```python
from build123d import *

# Parameters (mm, degrees)
SKETCH1_R               = 60
SKETCH1_R_2             = 2.5
SKETCH1_R_3             = 3
BOSS_EXTRUDE1_DEPTH     = 3
CUT_EXTRUDE1_DEPTH      = 85.905830189
CUT_EXTRUDE1_DEPTH_BACK = 85.905830189
SKETCH2_R               = 3


with BuildPart() as part:
    # Sketch1 → Boss-Extrude1 (new body)
    with BuildSketch(Plane(origin=(0, 0, 0), x_dir=(1, 0, 0), z_dir=(0, 1, 0))):
        with Locations(Location((0, 0, 0), (0, 0, 270))):
            Circle(SKETCH1_R)
        with Locations(Location((-24.748737342, -24.748737342, 0), (0, 0, 270))):
            Circle(SKETCH1_R_2, mode=Mode.SUBTRACT)
        with Locations(Location((24.748737342, -24.748737342, 0), (0, 0, 270))):
            Circle(SKETCH1_R_2, mode=Mode.SUBTRACT)
        with Locations(Location((24.748737342, 24.748737342, 0), (0, 0, 270))):
            Circle(SKETCH1_R_2, mode=Mode.SUBTRACT)
        with Locations(Location((-24.748737342, 24.748737342, 0), (0, 0, 270))):
            Circle(SKETCH1_R_2, mode=Mode.SUBTRACT)
        with Locations(Location((-25, -43.301270189, 0), (0, 0, 270))):
            Circle(SKETCH1_R_3, mode=Mode.SUBTRACT)
        with Locations(Location((25, -43.301270189, 0), (0, 0, 270))):
            Circle(SKETCH1_R_3, mode=Mode.SUBTRACT)
        with Locations(Location((50, 0, 0), (0, 0, 270))):
            Circle(SKETCH1_R_3, mode=Mode.SUBTRACT)
        with Locations(Location((25, 43.301270189, 0), (0, 0, 270))):
            Circle(SKETCH1_R_3, mode=Mode.SUBTRACT)
        with Locations(Location((-25, 43.301270189, 0), (0, 0, 270))):
            Circle(SKETCH1_R_3, mode=Mode.SUBTRACT)
        with Locations(Location((-50, 0, 0), (0, 0, 270))):
            Circle(SKETCH1_R_3, mode=Mode.SUBTRACT)
    extrude(amount=BOSS_EXTRUDE1_DEPTH)

    # Sketch2 → Cut-Extrude1 (cut, two sides: drawn at the far end of the back side and taken through both)
    with BuildSketch(Plane(origin=(0, 3, 0), x_dir=(1, 0, 0), z_dir=(0, 1, 0)).offset(-CUT_EXTRUDE1_DEPTH_BACK)):
        with Locations(Location((0, 0, 0), (0, 0, 270))):
            Circle(SKETCH2_R)
    extrude(amount=CUT_EXTRUDE1_DEPTH + CUT_EXTRUDE1_DEPTH_BACK, mode=Mode.SUBTRACT)


solid = part.part
```
The model under review builds one solid part; all positions refer to its coordinate system, in mm. Round coordinates to 2 decimals unless told otherwise and drop trailing zeros. Order: outer loops, then holes, each group sorted by start corner. A loop starts at its lowest first (then second) coordinate and runs counter-clockwise, first axis right, second up.
(1) Take a section at B-B, the plane y = 0.55. Count the separate pieces of the cut face and the enclosed holes in it, plus the area to 3 significant figures.
Working result:
separate pieces: 1
enclosed holes: 11
area: 11,000 mm2
(2) Take a section at A-A, the plane z = 0. State the section outline as (x, y) points, plus the area to 3 significant figures.
Working result:
outline: (-60, 0) - (-53, 0) - (-53, 3) - (-60, 3) - close; (-47, 0) - (-3, 0) - (-3, 3) - (-47, 3) - close; (3, 0) - (47, 0) - (47, 3) - (3, 3) - close; (53, 0) - (60, 0) - (60, 3) - (53, 3) - close
area: 306 mm2
(3) Take a section at C-C, the plane x = -50. State the section outline as (y, z) points.
Working result:
outline: (0, -33.17) - (3, -33.17) - (3, -3) - (0, -3) - close; (0, 3) - (3, 3) - (3, 33.17) - (0, 33.17) - close
(4) Mouldability with a two-part tool opening along Z and no side actions: class faces 1 (the face through (2.64, 1.48, -59.94)), 2 (the face through (-24.1, 1.48, -40.44)), 3 (the face through (1, 0, 12)) as released by +Z, released by -Z, zero draft, split by the parting line, or undercut.
Working result:
face 1: split by the parting line
face 2: undercut
face 3: zero draft
(5) Take a section at D-D, the plane x = 12. State the section outline as (y, z) points.
Working result:
outline: (0, -58.79) - (3, -58.79) - (3, 58.79) - (0, 58.79) - close
(6) Wall thickness on L1, parallel to Z at x = -25.5, y = 1.45; L2, parallel to Z at x = 22.5, y = 2.95; L3, parallel to Z at x = -27.5, y = 0.9: over which ranges is each line inside the solid? List them lowest first.
Working result:
L1: z = -54.31 to -46.26, -40.34 to -27.13, -22.36 to 22.36, 27.13 to 40.34, 46.26 to 54.31
L2: z = -55.62 to -44.96, -41.64 to -25.84, -23.66 to 23.66, 25.84 to 41.64, 44.96 to 55.62
L3: z = -53.33 to -44.96, -41.64 to 41.64, 44.96 to 53.33
